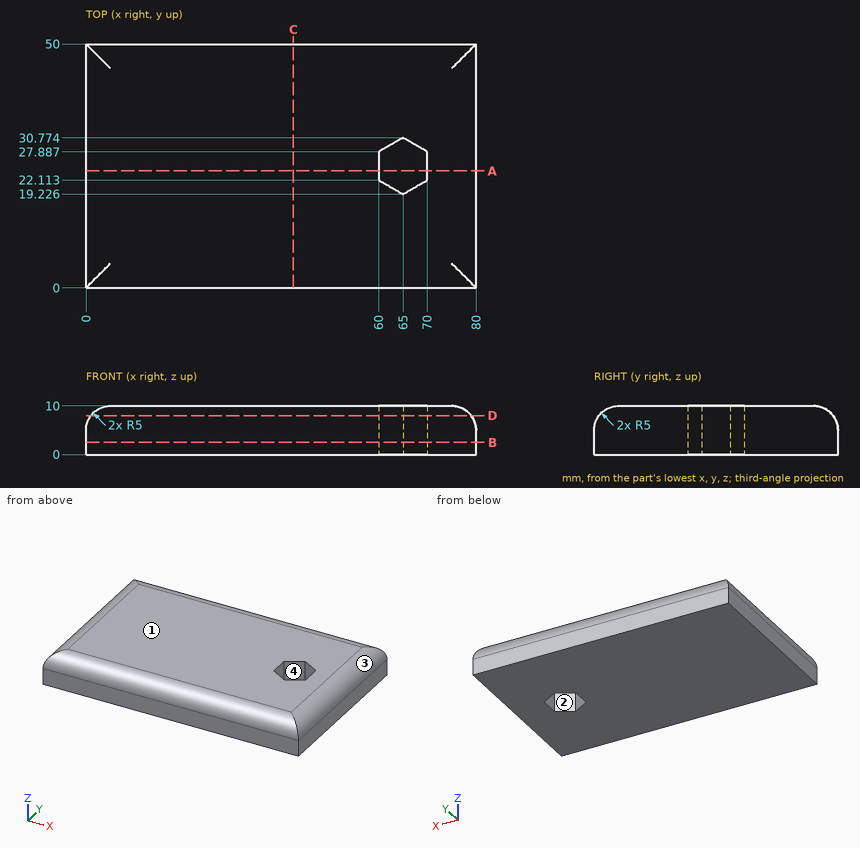
Verification items for this drawing (mm, ordinates from the low corner). Round coordinates to 2 decimals unless told otherwise and drop trailing zeros. Write each loop counter-clockwise with the first axis right and the second up, starting at its lowest first coordinate (ties: lowest second). Pieces come first, ordered by that corner, then holes. Notation, with made-up numbers: M 45.25,-36.5 L 70.25,-36.5 A23 cw 70.25,-28.5 Z; hole C 39.5,22 d9. An arc over 180 degrees is marked long. Write item = value, one per line. Start each with the question number.
1. Section check A-A, the plane y = 24. Record the cut outline in (x, z).
2. Section check D-D, the plane z = 8. Record the cut outline in (x, y).
3. Scan lines: line 1 (X direction, y = 25.5, z = 7.25) (1 decimal); line 2 (X direction, y = 20.5, z = 8) (1 decimal); line 3 (Y direction, x = 66.5, z = 5.75) (1 decimal). Record each from-to range of solid material in increasing order. Write a range as [from, to].
4. Release check for a two-part mould opening along X. For the marked faces 1, 2, 3 and 4 record: pulls with the +X half, pulls with the -X half, needs draft (parallel to the pull), parting line crosses it, or undercut.
5. Section check B-B, the plane z = 2.5. Record the cut outline in (x, y), then the cut area to 3 significant figures.
6. Gauge pin test, flat end, axial feed: pin 1 (10 mm diameter, centred on x = 15.5, y = 21, fed in from -Z). Record the tip position at first contact, or that the pin passes through.
7. Section check C-C, the plane x = 42.5. Record the cut outline in (y, z), then the cut area to 3 significant figures.
Results found:
q1.outline = M 0,0 L 60,0 L 60,10 L 5,10 A5 ccw 0,5 Z; M 70,0 L 80,0 L 80,5 A5 ccw 75,10 L 70,10 Z
q2.outline = M 1,1 L 79,1 L 79,49 L 1,49 Z; hole M 60,22.11 L 65,19.23 L 70,22.11 L 70,27.89 L 65,30.77 L 60,27.89 Z
q3.line_1 = [0.5, 60], [70, 79.5]
q3.line_2 = [1, 62.8], [67.2, 79]
q3.line_3 = [0.1, 20.1], [29.9, 49.9]
q4.face_1 = needs draft
q4.face_2 = undercut
q4.face_3 = pulls with the +X half
q4.face_4 = undercut
q5.outline = M 0,0 L 80,0 L 80,50 L 0,50 Z; hole M 60,22.11 L 65,19.23 L 70,22.11 L 70,27.89 L 65,30.77 L 60,27.89 Z
q5.area = 3,910 mm^2
q6.pin_1 = 0
q7.outline = M 0,0 L 50,0 L 50,5 A5 ccw 45,10 L 5,10 A5 ccw 0,5 Z
q7.area = 489 mm^2
